Design review of the part built by this model. Coordinates are the model's own, in mm. Coordinates: 2 decimals unless noted, no trailing zeros. Loops run counter-clockwise (first coordinate to the right, second up) from the corner with the lowest first, then second, coordinate; pieces in that order, holes last. Notation, with made-up numbers: (-37, 22.5) -> (17, 22.5) arc R26 cw to (17, 61.5) -> close; hole circle Ø8 at (51, 87.5). An arc over 180 degrees is marked (long way). Use a Markdown table: item, result. Add a question column.
Q1. Take a section at B-B on y = -0.65. Write out the cut boundary in (x, z).
Q2. Take a section at C-C on z = -2.5. Write out the cut boundary in (x, y).
Q3. Take a section at D-D on x = 5.75. Write out the cut boundary in (y, z), plus the area to 3 significant figures.
Q4. Draft analysis for pull direction X (two halves, no side actions). For faces 1 (the face through (8.5, 0, -0.1)), 2 (the face through (5.45, -0.02, 1.43)), 3 (the face through (-8.5, 0, 0.1)), state which applies: pulls with the +X half, pulls with the -X half, needs draft (parallel to the pull), parting line crosses it, or undercut.
Q5. Take a section at A-A on z = 0. Write out the cut boundary in (x, y).
Q6. Clearance check with a flat-ended pin moving along its axis: pin 1 Ø1 at (y, z) = (-0.5, 1.5) entering from -X. State where the tip first meets the part, or that it passes through.
Q7. For probe 1 along X at (y, z) = (-0.8, 0); probe 2 along X at (y, z) = (-1.05, 1); probe 3 along Z at (x, y) = (-3.75, -1.1), list the stretches that pass through material, from the lowest coordinate up.
from build123d import *

# Parameters (mm, degrees)
SKETCH1_R               = 1.5
BOSS_EXTRUDE1_DEPTH     = 1.5
CUT_EXTRUDE1_DEPTH      = 10.313968005
CUT_EXTRUDE1_DEPTH_BACK = 10.313968005
SKETCH2_W               = 7
SKETCH2_H               = 1.6
FILLET1_R               = 5
FILLET2_R               = 5


with BuildPart() as part:
    # Sketch1 → Boss-Extrude1 (new, symmetric)
    with BuildSketch(Plane(origin=(0, 0, 0), x_dir=(1, 0, 0), z_dir=(0, 1, 0))):
        with BuildLine():
            Line((-5, 3.5), (5, 3.5))
            ThreePointArc((5, 3.5), (8.5, 0), (5, -3.5))
            Line((5, -3.5), (-5, -3.5))
            ThreePointArc((-5, -3.5), (-8.5, 0), (-5, 3.5))
        make_face()
        with Locations(Location((-5, 0, 0), (0, 0, 270))):
            Circle(SKETCH1_R, mode=Mode.SUBTRACT)
        with Locations(Location((5, 0, 0), (0, 0, 270))):
            Circle(SKETCH1_R, mode=Mode.SUBTRACT)
    extrude(amount=BOSS_EXTRUDE1_DEPTH, both=True)

    # Sketch2 → Cut-Extrude1 (cut, two sides: drawn at the far end of the back side and taken through both)
    with BuildSketch(Plane(origin=(0, 0, 0), x_dir=(1, 0, 0), z_dir=(0, 1, 0)).offset(-CUT_EXTRUDE1_DEPTH_BACK)):
        with Locations((0, -2.7)):
            Rectangle(SKETCH2_W, SKETCH2_H)
        with Locations((0, 2.7)):
            Rectangle(SKETCH2_W, SKETCH2_H)
    extrude(amount=CUT_EXTRUDE1_DEPTH + CUT_EXTRUDE1_DEPTH_BACK, mode=Mode.SUBTRACT)

    # Fillet1
    # the kernel refuses this fillet: 5 mm, written as the material it adds along each edge
    with BuildSketch(Plane(origin=(-3.5, 1.5, 1.9), x_dir=(0, 0, 1), z_dir=(0, -1, 0)), Plane(origin=(3.5, 1.5, -1.9), x_dir=(0, 0, -1), z_dir=(0, -1, 0))) as fillet1_piece_1:
        with BuildLine():
            CenterArc((5, -3.666060556), FILLET1_R, 132.843643044, 47.156356956)
            Line((0, -3.666060556), (-0.1, -3.666060556))
            Line((-0.1, -3.666060556), (-0.1, 0))
            Line((-0.1, 0), (0, 0.1))
            ThreePointArc((0, 0.1), (0.8, 0.1), (1.532, 0.073321211))
            Line((1.532, 0.073321211), (1.6, 0))
        make_face()
    extrude(amount=3)
    with BuildSketch(Plane(origin=(-3.5, 1.5, -1.9), x_dir=(1, 0, 0), z_dir=(0, -1, 0))) as fillet1_piece_2:
        with BuildLine():
            CenterArc((3.666060556, -5), FILLET1_R, 90, 47.156356956)
            Line((0, -1.6), (-0.073321211, -1.532))
            ThreePointArc((-0.073321211, -1.532), (-0.1, -0.8), (-0.1, 0))
            Line((-0.1, 0), (0, 0.1))
            Line((0, 0.1), (3.666060556, 0.1))
            Line((3.666060556, 0.1), (3.666060556, 0))
        make_face()
    extrude(amount=3)
    with BuildSketch(Plane(origin=(3.5, -1.5, 1.9), x_dir=(-1, 0, 0), z_dir=(0, 1, 0))) as fillet1_piece_3:
        with BuildLine():
            CenterArc((3.666060556, 5), FILLET1_R, 222.843643044, 47.156356956)
            Line((0, 1.6), (-0.073321211, 1.532))
            ThreePointArc((-0.073321211, 1.532), (-0.1, 0.8), (-0.1, 0))
            Line((-0.1, 0), (0, -0.1))
            Line((0, -0.1), (3.666060556, -0.1))
            Line((3.666060556, -0.1), (3.666060556, 0))
        make_face()
    extrude(amount=3)

    # Fillet2
    # the kernel refuses this fillet: 5 mm, written as the material it takes off along each edge
    with BuildSketch(Plane(origin=(-3.5, 5.25, 3.5), x_dir=(0.7655176455574427, 0, -0.6434149006202682), z_dir=(0, -1, 0)), Plane(origin=(3.5, -5.25, 3.5), x_dir=(-0.7655176455574455, 0, -0.6434149006202647), z_dir=(0, 1, 0))) as fillet2_piece_1:
        with BuildLine():
            CenterArc((1.856470149, -4.961557983), FILLET2_R, 97.109423017, 29.828495219)
            Line((-1.148276468, -0.965122351), (0, 0))
            ThreePointArc((0, 0), (0.618823383, -0.038442017), (1.237646766, 0))
        make_face()
    extrude(amount=10.5, mode=Mode.SUBTRACT)
    with BuildSketch(Plane(origin=(-3.5, -5.25, -3.5), x_dir=(-1.0, 0, 2.909376443463916e-12), z_dir=(0, 1, 0))) as fillet2_piece_2:
        with BuildLine():
            CenterArc((1.771179679, 4.992640742), FILLET2_R, 237.062489078, 29.828495219)
            ThreePointArc((-0.947440439, 0.796320371), (-0.448986053, 0.427588228), (0, 0))
            Line((0, 0), (1.5, 0))
        make_face()
    extrude(amount=10.5, mode=Mode.SUBTRACT)
    with BuildSketch(Plane(origin=(3.5, -5.25, -3.5), x_dir=(-0.7655176455574453, 0, 0.6434149006202652), z_dir=(0, 1, 0))) as fillet2_piece_3:
        with BuildLine():
            CenterArc((1.856470149, 4.961557983), FILLET2_R, 233.062081764, 29.828495219)
            Line((-1.148276468, 0.965122351), (0, 0))
            ThreePointArc((0, 0), (0.618823383, 0.038442017), (1.237646766, 0))
        make_face()
    extrude(amount=10.5, mode=Mode.SUBTRACT)


solid = part.part
Answer list:
| question | item | result |
|---|---|---|
| 1 | outline | (-5, -3.5) arc R5 ccw to (-2.55, -2.7) arc R5 cw to (0, -1.9) arc R5 cw to (2.55, -2.7) arc R5 ccw to (5, -3.5) arc R3.5 ccw to (5, 3.5) arc R5 ccw to (2.55, 2.7) arc R5 cw to (0, 1.9) arc R5 cw to (-2.55, 2.7) arc R5 ccw to (-5, 3.5) arc R3.5 ccw to start; hole circle Ø3 at (-5, 0); hole circle Ø3 at (5, 0) |
| 2 | outline | (-7.45, -1.5) -> (-2.21, -1.5) -> (-2.21, 1.5) -> (-7.45, 1.5) -> close; (2.21, -1.5) -> (7.45, -1.5) -> (7.45, 1.5) -> (2.21, 1.5) -> close |
| 3 | outline | (-1.5, -3.42) -> (1.5, -3.42) -> (1.5, -1.3) -> (-1.5, -1.3) -> close; (-1.5, 1.3) -> (1.5, 1.3) -> (1.5, 3.42) -> (-1.5, 3.42) -> close |
| 3 | area | 12.7 mm² |
| 4 | face 1 | pulls with the +X half |
| 4 | face 2 | undercut |
| 4 | face 3 | pulls with the -X half |
| 5 | outline | (-8.5, -1.5) -> (-6.5, -1.5) -> (-6.5, 1.5) -> (-8.5, 1.5) -> close; (-3.5, -1.5) -> (3.5, -1.5) -> (3.5, 1.5) -> (-3.5, 1.5) -> close; (6.5, -1.5) -> (8.5, -1.5) -> (8.5, 1.5) -> (6.5, 1.5) -> close |
| 6 | pin 1 | x = -8.35 |
| 7 | probe 1 | -8.5 to -6.5, -3.5 to 3.5, 6.5 to 8.5 |
| 7 | probe 2 | -8.35 to -6.12, -3.88 to 3.88, 6.12 to 8.35 |
| 7 | probe 3 | -3.27 to -0.83, 0.83 to 3.27 |
